from build123d import *

# Parameters (mm, degrees)
SKETCH1_W               = 20
SKETCH1_H               = 30
BOSS_EXTRUDE1_DEPTH     = 5
SKETCH2_R               = 10
SKETCH2_R_2             = 8.125
BOSS_EXTRUDE2_DEPTH     = 15
CUT_EXTRUDE3_DEPTH      = 24.452078799
CUT_EXTRUDE3_DEPTH_BACK = 24.452078799
SKETCH5_R               = 8.125
SKETCH3_R               = 1.75
CUT_EXTRUDE1_DEPTH      = 5
CHAMFER1_SIZE           = 1
CUT_EXTRUDE2_DEPTH      = 27.925824036
CUT_EXTRUDE2_DEPTH_BACK = 27.925824036
SKETCH4_R               = 1.75


with BuildPart() as part:
    # Sketch1 → Boss-Extrude1 (new body)
    with BuildSketch(Plane(origin=(0, 0, 0), x_dir=(1, 0, 0), z_dir=(0, 1, 0))):
        Rectangle(SKETCH1_W, SKETCH1_H)
    extrude(amount=BOSS_EXTRUDE1_DEPTH)

    # Sketch2 → Boss-Extrude2 (add)
    with BuildSketch(Plane(origin=(0, 5, 0), x_dir=(1, 0, 0), z_dir=(0, 1, 0))):
        with Locations(Location((0, 0, 0), (0, 0, 180))):
            Circle(SKETCH2_R)
        with Locations(Location((0, 0, 0), (0, 0, 270))):
            Circle(SKETCH2_R_2, mode=Mode.SUBTRACT)
    extrude(amount=BOSS_EXTRUDE2_DEPTH)

    # Sketch5 → Cut-Extrude3 (cut, two sides: drawn at the far end of the back side and taken through both)
    with BuildSketch(Plane(origin=(0, 5, 0), x_dir=(1, 0, 0), z_dir=(0, 1, 0)).offset(-CUT_EXTRUDE3_DEPTH_BACK)):
        with Locations(Location((0, 0, 0), (0, 0, 270))):
            Circle(SKETCH5_R)
    extrude(amount=CUT_EXTRUDE3_DEPTH + CUT_EXTRUDE3_DEPTH_BACK, mode=Mode.SUBTRACT)

    # Sketch3 → Cut-Extrude1 (cut)
    with BuildSketch(Plane(origin=(0, 5, 0), x_dir=(1, 0, 0), z_dir=(0, 1, 0))):
        with Locations(Location((-5, 12, 0), (0, 0, 270))):
            Circle(SKETCH3_R)
        with Locations(Location((5, 12, 0), (0, 0, 270))):
            Circle(SKETCH3_R)
        with Locations(Location((5, -12, 0), (0, 0, 270))):
            Circle(SKETCH3_R)
        with Locations(Location((-5, -12, 0), (0, 0, 270))):
            Circle(SKETCH3_R)
    extrude(amount=-CUT_EXTRUDE1_DEPTH, mode=Mode.SUBTRACT)

    # Chamfer1
    chamfer1_edges = [part.edges().sort_by_distance(p)[0] for p in [
        (0, 20, -8.125),
    ]]
    chamfer(chamfer1_edges, length=CHAMFER1_SIZE)

    # Sketch4 → Cut-Extrude2 (cut, two sides: drawn at the far end of the back side and taken through both)
    with BuildSketch(Plane(origin=(0, 0, 0), x_dir=(0, 0, -1), z_dir=(1, 0, 0)).offset(-CUT_EXTRUDE2_DEPTH_BACK)):
        with Locations((0, 12.5)):
            Circle(SKETCH4_R)
    extrude(amount=CUT_EXTRUDE2_DEPTH + CUT_EXTRUDE2_DEPTH_BACK, mode=Mode.SUBTRACT)


solid = part.part
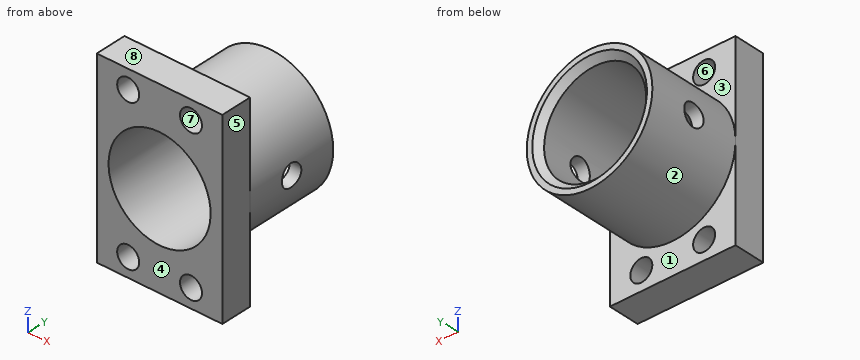
The model under review builds one solid part; all positions refer to its coordinate system, in mm. Face numbers are marked on the shaded views. A direction names the side the tool comes from. Round coordinates to 2 decimals unless told otherwise and drop trailing zeros. Loops run counter-clockwise (first coordinate to the right, second up) from the corner with the lowest first, then second, coordinate; pieces in that order, holes last. Notation, with made-up numbers: (9.5, 34) -> (52.5, 34) arc R32 cw to (52.5, 60) -> close; hole circle Ø3 at (23.25, 43.5). An arc over 180 degrees is marked (long way). Write item = value, one per line. Start each with the question number.
Item 1: Insertion check: pin 1 (4.5 mm diameter, centred on x = -1.5, z = -6, fed in from +Y); pin 2 (4.5 mm diameter, centred on y = 12.5, z = 0, fed in from -X); pin 3 (7.5 mm diameter, centred on x = 3.5, z = 4, fed in from +Y); pin 4 (6 mm diameter, centred on y = 17, z = 5.5, fed in from -X). Each pin has a flat end and moves straight along its axis. Give the tip position at first contact, or say it passes through.
Item 2: Mouldability with a two-part tool opening along Z and no side actions: class the marked faces 5, 6, 7 and 8 as released by +Z, released by -Z, zero draft, split by the parting line, or undercut.
Item 3: Take a section at C-C on x = 0. Give the boundary of the cut face in (y, z) (3 decimals), plus the area to 3 significant figures.
Item 4: Take a section at B-B on z = 12. Give the boundary of the cut face in (x, y).
Item 5: For the marked faces 1, 2, 3 and 4, list the 3-axis set-ups (+Z, -Z, +X, -X, +Y, -Y) from which the entire face can be reached by the end or side of a thin tool; tool diameter is ignored.
Item 6: Take a section at D-D on y = 12.5. Give the boundary of the cut face in (x, z) (3 decimals).
Item 7: Take a section at A-A on y = 1. Give the boundary of the cut face in (x, z) (3 decimals), plus the area to 3 significant figures.
Item 8: To check wall thickness, follow L1, parallel to X at y = 1.25, z = -12; L2, parallel to Z at x = 0.25, y = 8.5; L3, parallel to Z at x = 3.5, y = 2. State the ranges of each line that lie inside material, in increasing order.
Result:
q1.pin_1 = 19.31
q1.pin_2 = -10
q1.pin_3 = 19.94
q1.pin_4 = -9.68
q2.face_5 = zero draft
q2.face_6 = undercut
q2.face_7 = undercut
q2.face_8 = released by +Z
q3.outline = (0, -15) -> (5, -15) -> (5, -10) -> (20, -10) -> (20, -9.125) -> (19, -8.125) -> (0, -8.125) -> close; (0, 8.125) -> (19, 8.125) -> (20, 9.125) -> (20, 10) -> (5, 10) -> (5, 15) -> (0, 15) -> close
q3.area = 124 mm²
q4.outline = (-10, 0) -> (-6.75, 0) -> (-6.75, 5) -> (-10, 5) -> close; (-3.25, 0) -> (3.25, 0) -> (3.25, 5) -> (-3.25, 5) -> close; (6.75, 0) -> (10, 0) -> (10, 5) -> (6.75, 5) -> close
q5.face_1 = -Z, +Y
q5.face_2 = +Y
q5.face_3 = +Z, +Y
q5.face_4 = +Z, -Z, +X, -X, -Y
q6.outline = (-9.846, -1.75) arc R10 ccw to (9.846, -1.75) -> (7.934, -1.75) arc R8.125 cw to (-7.934, -1.75) -> close; (-9.846, 1.75) -> (-7.934, 1.75) arc R8.125 cw to (7.934, 1.75) -> (9.846, 1.75) arc R10 ccw to start
q7.outline = (-10, -15) -> (10, -15) -> (10, 15) -> (-10, 15) -> close; hole circle Ø16.25 at (0, 0); hole circle Ø3.5 at (-5, -12); hole circle Ø3.5 at (-5, 12); hole circle Ø3.5 at (5, -12); hole circle Ø3.5 at (5, 12)
q7.area = 354 mm²
q8.L1 = -10 to -6.75, -3.25 to 3.25, 6.75 to 10
q8.L2 = -10 to -8.12, 8.12 to 10
q8.L3 = -15 to -12.9, -11.1 to -7.33, 7.33 to 11.1, 12.9 to 15
